Input: part model. Units: mm. Frame: model coordinates. A direction names the side the tool comes from. Coordinates: 2 decimals unless noted, no trailing zeros. Write each loop counter-clockwise with the first axis right and the second up, starting at its lowest first coordinate (ties: lowest second). Pieces come first, ordered by that corner, then holes.
from build123d import *

# Parameters (mm, degrees)
CROQUIS1_R              = 100
SALIENTE_EXTRUIR1_DEPTH = 3
CROQUIS3_R              = 110
CORTAR_EXTRUIR1_DEPTH   = 3
REDONDEO1_R             = 10
CORTAR_EXTRUIR3_DEPTH   = 10
CROQUIS10_R             = 1.5
CORTAR_EXTRUIR4_DEPTH   = 142.453172607
CROQUIS11_R             = 2
CROQUIS11_W             = 17
CROQUIS11_H             = 50
CROQUIS11_W_2           = 38
CROQUIS11_H_2           = 40
CORTAR_EXTRUIR5_DEPTH   = 10
REDONDEO2_R             = 3
CROQUIS12_R             = 1.5
CORTAR_EXTRUIR6_DEPTH   = 142.453172607


with BuildPart() as part:
    # Croquis1 → Saliente-Extruir1 (new body)
    with BuildSketch(Plane.XY):
        Circle(CROQUIS1_R)
    extrude(amount=SALIENTE_EXTRUIR1_DEPTH)

    # Croquis3 → Cortar-Extruir1 (cut)
    with BuildSketch(Plane.XY.offset(3)):
        with Locations((190, 0)):
            Circle(CROQUIS3_R)
    extrude(amount=-CORTAR_EXTRUIR1_DEPTH, mode=Mode.SUBTRACT)

    # Redondeo1
    redondeo1_edges = [part.edges().sort_by_distance(p)[0] for p in [
        (89.473684211, -44.659375654, 1.5),
        (89.473684211, 44.659375654, 1.5),
    ]]
    fillet(redondeo1_edges, radius=REDONDEO1_R)

    # Croquis7 → Cortar-Extruir3 (cut)
    with BuildSketch(Plane.XY.offset(3)):
        Polygon((-71.939339828, -40.119534675), (-40.119534675, -71.939339828), (-57.797204204, -89.617009358), (-89.617009358, -57.797204204), align=None)
        Polygon((-40.119534675, 71.939339828), (-71.939339828, 40.119534675), (-89.617009358, 57.797204204), (-57.797204204, 89.617009358), align=None)
        Polygon((71.939339828, 40.119534675), (40.119534675, 71.939339828), (57.797204204, 89.617009358), (89.617009358, 57.797204204), align=None)
        Polygon((40.119534675, -71.939339828), (71.939339828, -40.119534675), (89.617009358, -57.797204204), (57.797204204, -89.617009358), align=None)
    extrude(amount=-CORTAR_EXTRUIR3_DEPTH, mode=Mode.SUBTRACT)

    # Croquis10 → Cortar-Extruir4 (cut, through all)
    with BuildSketch(Plane.XY.offset(3)):
        with Locations((-20, 8.5)):
            Circle(CROQUIS10_R)
        with Locations((14.74, 72.95)):
            Circle(CROQUIS10_R)
        with Locations((-25.9, 72.95)):
            Circle(CROQUIS10_R)
        with Locations(Location((14.74, -72.95, 0), (0, 0, 180))):
            Circle(CROQUIS10_R)
        with Locations(Location((-25.9, -72.95, 0), (0, 0, 180))):
            Circle(CROQUIS10_R)
    extrude(amount=-CORTAR_EXTRUIR4_DEPTH, mode=Mode.SUBTRACT)

    # Croquis11 → Cortar-Extruir5 (cut)
    with BuildSketch(Plane.XY.offset(3)):
        with Locations((0, 92)):
            Circle(CROQUIS11_R)
        with Locations((0, -92)):
            Circle(CROQUIS11_R)
        with Locations((72, 31.694913472)):
            Circle(CROQUIS11_R)
        with Locations((72, -31.694913472)):
            Circle(CROQUIS11_R)
        with Locations((-85, -30)):
            Circle(CROQUIS11_R)
        with Locations((-85, 30)):
            Circle(CROQUIS11_R)
        with Locations((65.5, 0)):
            Rectangle(CROQUIS11_W, CROQUIS11_H)
        Polygon((55.443488939, 35.561561695), (24.824867154, 66.18018348), (13.617673752, 24.354368293), align=None)
        Polygon((13.617673752, -24.354368293), (55.443488939, -35.561561695), (24.824867154, -66.18018348), align=None)
        with Locations((-56, 0)):
            Rectangle(CROQUIS11_W_2, CROQUIS11_H_2)
    extrude(amount=-CORTAR_EXTRUIR5_DEPTH, mode=Mode.SUBTRACT)

    # Redondeo2
    redondeo2_edges = [part.edges().sort_by_distance(p)[0] for p in [
        (74, 25, 1.5),
        (74, -25, 1.5),
        (57, -25, 1.5),
        (57, 25, 1.5),
        (55.443488939, 35.561561695, 1.5),
        (13.617673752, 24.354368293, 1.5),
        (24.824867154, 66.18018348, 1.5),
        (24.824867154, -66.18018348, 1.5),
        (13.617673752, -24.354368293, 1.5),
        (55.443488939, -35.561561695, 1.5),
        (-37, 20, 1.5),
        (-37, -20, 1.5),
        (-75, -20, 1.5),
        (-75, 20, 1.5),
    ]]
    fillet(redondeo2_edges, radius=REDONDEO2_R)

    # Croquis12 → Cortar-Extruir6 (cut, through all)
    with BuildSketch(Plane(origin=(0, 0, 0), x_dir=(-1, 0, 0), z_dir=(0, 0, -1))):
        with Locations((-19, 22)):
            Circle(CROQUIS12_R)
        with Locations((-19, -22)):
            Circle(CROQUIS12_R)
    extrude(amount=-CORTAR_EXTRUIR6_DEPTH, mode=Mode.SUBTRACT)


solid = part.part
Item 1: Access query for faces 1 (the face through (46.64, -78.46, 1.52)), 2 (the face through (-78.28, 46.46, 1.52)), 3 (the face through (34.31, -29.9, 1.52)), 4 (the face through (78.28, -46.46, 1.52)). Directions: +Z, -Z, +X, -X, +Y, -Y. A direction counts if a zero-diameter tool reaches every point of the face in a straight line with its end or side. Return the directions, or none.
Item 2: Material intervals for line 1 (X direction, y = -2, z = 0.7); line 2 (X direction, y = -72.95, z = 2.15); line 3 (Y direction, x = -42.5, z = 2.8), sorted ascending.
Item 3: Pull-direction query (X, two-part tool) for faces 5 (the face through (-46.64, 78.46, 1.52)), 6 (the face through (40.297, -50.708, 1.521)), 7 (the face through (-7, 1, 3)); classes: released by +X, released by -X, zero draft, split by the parting line, or undercut.
Item 4: Section query C-C, the plane x = 46.5. Return loops of the section in (y, z), then the cut area to 3 significant figures.
Item 5: Section query B-B, the plane x = -58. Return loops of the section in (y, z).
Item 6: Pin query (flat end, axial travel): pin 1 Ø3 at (x, y) = (0, 92) entering from -Z; pin 2 Ø1 at (x, z) = (28.5, 2) entering from -Y; pin 3 Ø1 at (x, z) = (61, 1.5) entering from -Y; pin 4 Ø0.9 at (y, z) = (-5.5, 1) entering from -X. Return the tip coordinate at first contact, or that it passes through.
Item 7: Section query A-A, the plane y = 13.5. Return loops of the section in (x, z).
Item 8: Section query D-D, the plane z = 2.15. State how many separate pieces and enclosed holes the cut face has, then the cut area to 3 significant figures.
The answers:
1. face 1: +Z, -Z, +X
1. face 2: +Z, -Z, +Y
1. face 3: +Z, -Z
1. face 4: +Z, -Z, -Y
2. line 1: x = -99.98 to -75, -37 to 57, 74 to 80.02
2. line 2: x = -41.13 to -27.4, -24.4 to 13.24, 16.24 to 41.13
2. line 3: y = -90.52 to -74.32, -69.56 to -20, 20 to 69.56, 74.32 to 90.52
3. face 5: released by -X
3. face 6: undercut
3. face 7: zero draft
4. outline: (-88.53, 0) - (-78.32, 0) - (-78.32, 3) - (-88.53, 3) - close; (-65.56, 0) - (-44.51, 0) - (-44.51, 3) - (-65.56, 3) - close; (-33.17, 0) - (33.17, 0) - (33.17, 3) - (-33.17, 3) - close; (44.51, 0) - (65.56, 0) - (65.56, 3) - (44.51, 3) - close; (78.32, 0) - (88.53, 0) - (88.53, 3) - (78.32, 3) - close
4. area: 387 mm2
5. outline: (-54.06, 0) - (-20, 0) - (-20, 3) - (-54.06, 3) - close; (20, 0) - (54.06, 0) - (54.06, 3) - (20, 3) - close
6. pin 1: passes through
6. pin 2: stops at y = -96
6. pin 3: stops at y = -51.56
6. pin 4: stops at x = -99.87
7. outline: (-99.08, 0) - (-75, 0) - (-75, 3) - (-99.08, 3) - close; (-37, 0) - (57, 0) - (57, 3) - (-37, 3) - close; (74, 0) - (80.83, 0) - (80.83, 3) - (74, 3) - close
8. separate pieces: 1
8. enclosed holes: 17
8. area: 22,600 mm2
